```python
from build123d import *

# Parameters (mm, degrees)
BOSS_EXTRUDE1_DEPTH = 9.899999946


with BuildPart() as part:
    # Sketch1 → Boss-Extrude1 (new body)
    with BuildSketch(Plane(origin=(0, 0, 0), x_dir=(-1, 0, 0), z_dir=(0, 0, -1))):
        Polygon((30.050000664, 0), (30.050000664, 9.973500704), (25.049001075, 9.973500704), (25.049001075, 10.000000559), (25.001000706, 10.000000559), (25.001000706, 9.974000824), (19.949001889, 9.974000824), (19.949001889, 20.025999921), (25.001000706, 20.025999921), (25.001000706, 20.000001118), (25.050001316, 20.000001118), (25.050001316, 15.026001504), (30.050000664, 15.026001504), (30.050000664, 25.000002328), (5.050000664, 25.000002328), (5.050000664, 15.026001504), (9.999000318, 15.026001504), (9.999000318, 20.025999921), (15.051501118, 20.025999921), (15.051501118, 9.973500704), (10.051000718, 9.973500704), (5.050000664, 9.973500704), (5.050000664, 0), (15.024001023, 0), (15.024001023, 5.026000479), (20.076501822, 5.026000479), (20.076501822, 0), align=None)
    extrude(amount=-BOSS_EXTRUDE1_DEPTH)


solid = part.part
```
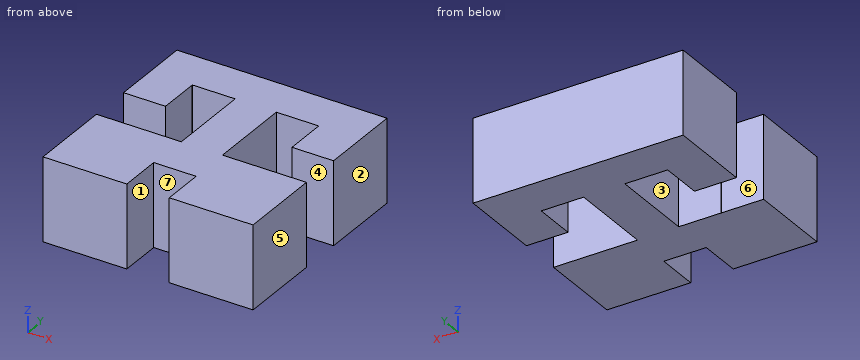
Input: part model. Units: mm. Frame: model coordinates. Face numbers are marked on the shaded views. A direction names the side the tool comes from. Coordinates: 2 decimals unless noted, no trailing zeros. Loops run counter-clockwise (first coordinate to the right, second up) from the corner with the lowest first, then second, coordinate; pieces in that order, holes last. Notation, with made-up numbers: (43, 81.5) - (94, 81.5) arc R22 cw to (94, 111.5) - close; hole circle Ø11 at (-31, 78). An arc over 180 degrees is marked (long way). Answer in a Markdown table with one row per item.
(1) Mould query, pull axis X, two halves, no side actions, for the marked faces 5, 6 and 7. Classes: pulls with the +X half, pulls with the -X half, needs draft (parallel to the pull), parting line crosses it, or undercut.
Model answer:
| item | result |
|---|---|
| face 5 | pulls with the +X half |
| face 6 | needs draft |
| face 7 | undercut |
(2) Set-up query: the marked faces 1, 2, 3 and 4. Return all of +Z, -Z, +X, -X, +Y, -Y with unobstructed straight access to the full face (end or side cutting, diameter ignored); none if empty.
Model answer:
| item | result |
|---|---|
| face 1 | +Z, -Z, -Y |
| face 2 | +Z, -Z, +X, +Y, -Y |
| face 3 | +Z, -Z |
| face 4 | +Z, -Z, +X |
(3) Cut plane B-B on y = 16.5. Output: boundary loops of the cut face in (x, z), plus the area to 3 significant figures.
Model answer:
| item | result |
|---|---|
| outline | (-30.05, 0) - (-25.05, 0) - (-25.05, 9.9) - (-30.05, 9.9) - close; (-19.95, 0) - (-15.05, 0) - (-15.05, 9.9) - (-19.95, 9.9) - close; (-10, 0) - (-5.05, 0) - (-5.05, 9.9) - (-10, 9.9) - close |
| area | 147 mm² |
(4) Cut plane C-C on y = 3.25. Output: boundary loops of the cut face in (x, z).
Model answer:
| item | result |
|---|---|
| outline | (-30.05, 0) - (-20.08, 0) - (-20.08, 9.9) - (-30.05, 9.9) - close; (-15.02, 0) - (-5.05, 0) - (-5.05, 9.9) - (-15.02, 9.9) - close |
(5) Cut plane A-A on x = -26. Output: boundary loops of the cut face in (y, z).
Model answer:
| item | result |
|---|---|
| outline | (0, 0) - (9.97, 0) - (9.97, 9.9) - (0, 9.9) - close; (15.03, 0) - (25, 0) - (25, 9.9) - (15.03, 9.9) - close |
(6) Material intervals for L1, parallel to X at y = 18, z = 4; L2, parallel to Y at x = -23.5, z = 2.5; L3, parallel to Y at x = -27.25, z = 5, sorted ascending. Write a range as from..to.
Model answer:
| item | result |
|---|---|
| L1 | x = -30.05..-25.05, -19.95..-15.05, -10..-5.05 |
| L2 | y = 0..9.97, 20.03..25 |
| L3 | y = 0..9.97, 15.03..25 |
